Autodesk Inventor part; units mm, degrees
ref_plane "YZ Plane" through (0, 0, 0) normal (1, 0, 0) x (0, 1, 0)
ref_plane "XZ Plane" through (0, 0, 0) normal (0, 1, 0) x (-1, 0, 0)
ref_plane "XY Plane" through (0, 0, 0) normal (0, 0, 1) x (1, 0, 0)
sketch "Sketch1" plane through (0, 0, 0) normal (0, 1, 0) x (-1, 0, 0)
  circle A0 centre (0, 0) radius 3
  dimension "d0" = 6
extrude "Extrusion1" add sketch "Sketch1" against normal blind 3
sketch "Sketch2" plane through (0, -3, 0) normal (0, -1, 0) x (1, 0, 0)
  circle A0 centre (0, 0) radius 1.5
  dimension "d3" = 3
extrude "Extrusion2" add sketch "Sketch2" along normal blind 12
sketch "Sketch3" plane through (0, 0, 0) normal (0, 1, 0) x (1, 0, 0)
  circle A0 centre (0, 0) radius 1.5 construction
  line L0 (1.4434, 0) -> (0.7217, -1.25)
  line L1 (0.7217, -1.25) -> (-0.7217, -1.25)
  line L2 (-0.7217, -1.25) -> (-1.4434, 0)
  line L3 (-1.4434, 0) -> (-0.7217, 1.25)
  line L4 (-0.7217, 1.25) -> (0.7217, 1.25)
  line L5 (0.7217, 1.25) -> (1.4434, 0)
  dimension "d8" = 2.5
extrude "Extrusion3" cut sketch "Sketch3" against normal blind 1.5
chamfer "Chamfer1" distance 0.25 angle 45 1 edges at (-1.5, -15, 0)
fillet "Fillet1" radius 0.25 2 edges at (3, 0, 0) (3, -3, 0)
chamfer "Chamfer2" distance 0.1 angle 45 6 edges at (0, 0, -1.25) (1.0825, 0, -0.625) (1.0825, 0, 0.625) (0, 0, 1.25) (-1.0825, 0, 0.625) (-1.0825, 0, -0.625)
thread "Thread2"
properties part number "M3-12" material "Steel, Carbon"
Input: part model. Units: mm. Frame: model coordinates. A direction names the side the tool comes from. Give positions to 0.01 mm unless a question says otherwise; leave off trailing zeros. Write each loop counter-clockwise with the first axis right and the second up, starting at its lowest first coordinate (ties: lowest second). Pieces come first, ordered by that corner, then holes. Notation, with made-up numbers: (-10, 84) - (48, 84) arc R22 ccw to (48, 107) - close; hole circle Ø1 at (73.5, 74.5). An arc over 180 degrees is marked (long way). Write item = value, one per line. Start each with the question number.
1) Material intervals for L1, parallel to Y at x = 0.5, z = -0.5; L2, parallel to Y at x = -1.25, z = 1.25; L3, parallel to Z at x = -1.25, y = -2.75, sorted ascending. Write a range as [from, to].
2) Pin query (flat end, axial travel): pin 1 (1.5 mm diameter, centred on x = 2, y = -9, fed in from -Z); pin 2 (2 mm diameter, centred on x = -2, z = -2, fed in from -Y); pin 3 (2 mm diameter, centred on y = -2.5, z = 2, fed in from -X). Return the tip coordinate at first contact, or that it passes through.
3) Cut plane B-B (y = -13.5). Return loops of the section in (x, z), and give its area (3 significant figures).
4) Draft query along Z for faces 4 (the face through (1.088, -0.79, 0.616)), 5 (the face through (0, -15, 0)), 6 (the face through (3, -1, 0)). Return one class per face: pulls with the +Z half, pulls with the -Z half, needs draft (parallel to the pull), parting line crosses it, or undercut.
5) Cut plane A-A (x = 0). Return loops of the section in (y, z).
6) Reachability of faces 1 (the face through (-1.2, 0, -1.2)), 2 (the face through (0, -1, -1.25)), 3 (the face through (-1.5, -8.79, -0.07)) from +Z, -Z, +X, -X, +Y, -Y: full face, straight path, thin tool, end or side. Return the list, or none.
Answers follow:
q1.L1 = [-15, -1.5]
q1.L2 = [-3, 0]
q1.L3 = [-2.73, 2.73]
q2.pin_1 = -0.83
q2.pin_2 = -3
q2.pin_3 = -2.83
q3.outline = circle Ø3 at (0, 0)
q3.area = 7.07 mm^2
q4.face_4 = undercut
q4.face_5 = needs draft
q4.face_6 = parting line crosses it
q5.outline = (-15, -1.25) - (-14.75, -1.5) - (-3, -1.5) - (-3, -2.75) arc R0.25 ccw to (-2.75, -3) - (-0.25, -3) arc R0.25 ccw to (0, -2.75) - (0, -1.35) - (-0.1, -1.25) - (-1.5, -1.25) - (-1.5, 1.25) - (-0.1, 1.25) - (0, 1.35) - (0, 2.75) arc R0.25 ccw to (-0.25, 3) - (-2.75, 3) arc R0.25 ccw to (-3, 2.75) - (-3, 1.5) - (-14.75, 1.5) - (-15, 1.25) - close
q6.face_1 = +Z, -Z, +X, -X, +Y
q6.face_2 = +Y
q6.face_3 = -Y
